Geometry: final body of the model. Coordinates: model frame, mm. Face numbers are marked on the shaded views. A direction names the side the tool comes from. Give positions to 0.01 mm unless a question says otherwise; leave off trailing zeros. Loops run counter-clockwise (first coordinate to the right, second up) from the corner with the lowest first, then second, coordinate; pieces in that order, holes last. Notation, with made-up numbers: (-15, 65.25) -> (19, 65.25) arc R14 cw to (19, 75.25) -> close; hole circle Ø8 at (16.5, 80). An arc over 180 degrees is marked (long way). Answer in a Markdown table with one row per item. Add a question column.
1) Section query B-B (z = 9.5). Return the cut outline in (x, y), plus the area to 3 significant figures.
2) Section query A-A (y = -1.5). Return the cut outline in (x, z).
3) Section query D-D (y = 8.75). Return the cut outline in (x, z).
4) Access query for the marked faces 5 and 6. Directions: +Z, -Z, +X, -X, +Y, -Y. A direction counts if a zero-diameter tool reaches every point of the face in a straight line with its end or side. Return the directions, or none.
5) Draft query along Y for the marked faces 1, 2, 3 and 4. Return one class per face: +Y half, -Y half, draft (parallel to the pull), parting line (faces both ways), or undercut.
6) Line query: line 1 (Y direction, x = 6.5, z = 14.25); line 2 (Y direction, x = -8.4, z = 5); line 3 (X direction, y = 4, z = 13). Output: solid intervals per line, ascending. Write a range as from..to.
7) First-contact query: P1, Ø0.9, axis at y = -5.5, z = 10, coming from the +X side; P2, Ø4.5, axis at y = 5, z = 15, coming from the +X side; P3, Ø6, axis at x = 8.5, y = 4.5, coming from the -Z side; P4, Ø8, axis at x = 0.5, z = 13.5, coming from the +Y side. Flat tips, straight axial feed; report the tip coordinate or a pass-through.
8) Section query C-C (y = -4.75). Return the cut outline in (x, z), plus the area to 3 significant figures.
```python
from build123d import *

# Parameters (mm, degrees)
SKETCH2_W           = 40
SKETCH2_H           = 20
BOSS_EXTRUDE2_DEPTH = 20
SKETCH3_W           = 20
SKETCH3_H           = 20
CUT_EXTRUDE1_DEPTH  = 10
SKETCH4_W           = 18.496290815
SKETCH4_H           = 3
CUT_EXTRUDE2_DEPTH  = 31
SKETCH5_R           = 1.5
CUT_EXTRUDE3_DEPTH  = 34.541019662
SKETCH8_R           = 1.5
CUT_EXTRUDE4_DEPTH  = 2.5
CUT_EXTRUDE6_DEPTH  = 31.347981811


with BuildPart() as part:
    # Sketch2 → Boss-Extrude2 (new body)
    with BuildSketch(Plane.XY):
        Rectangle(SKETCH2_W, SKETCH2_H)
    extrude(amount=BOSS_EXTRUDE2_DEPTH)

    # Sketch3 → Cut-Extrude1 (cut)
    with BuildSketch(Plane.ZY.offset(20)):
        with Locations((10, 0)):
            Rectangle(SKETCH3_W, SKETCH3_H)
    extrude(amount=-CUT_EXTRUDE1_DEPTH, mode=Mode.SUBTRACT)

    # Sketch4 → Cut-Extrude2 (cut, through all)
    with BuildSketch(Plane.XY.offset(20)):
        Polygon((-5, -1), (20, -1), (20, 0), (20, 10), (-5, 10), align=None)
        with Locations((10.751854593, -5.5)):
            Rectangle(SKETCH4_W, SKETCH4_H)
    extrude(amount=-CUT_EXTRUDE2_DEPTH, mode=Mode.SUBTRACT)

    # Sketch5 → Cut-Extrude3 (cut, through all)
    with BuildSketch(Plane(origin=(-5, 0, 0), x_dir=(0, 0, -1), z_dir=(1, 0, 0))):
        with Locations((-15.023649692, 4.5)):
            Circle(SKETCH5_R)
        with Locations((-5, 4.5)):
            Circle(SKETCH5_R)
    extrude(amount=-CUT_EXTRUDE3_DEPTH, mode=Mode.SUBTRACT)

    # Sketch8 → Cut-Extrude4 (cut)
    # profile 1 of 2: a face of its own
    with BuildSketch(Plane(origin=(-5, 0, 0), x_dir=(0, 0, -1), z_dir=(1, 0, 0))):
        Polygon((-12.208649692, 2.874758992), (-12.208649692, 6.125241008), (-15.023649692, 7.750482016), (-17.838649692, 6.125241008), (-17.838649692, 2.874758992), (-15.023649692, 1.249517984), align=None)
        with Locations((-15.023649692, 4.5)):
            Circle(SKETCH8_R, mode=Mode.SUBTRACT)
    # profile 2 of 2: a face of its own
    with BuildSketch(Plane(origin=(-5, 0, 0), x_dir=(0, 0, -1), z_dir=(1, 0, 0))):
        Polygon((-2.185, 2.874758992), (-2.185, 6.125241008), (-5, 7.750482016), (-7.815, 6.125241008), (-7.815, 2.874758992), (-5, 1.249517984), align=None)
        with Locations((-5, 4.5)):
            Circle(SKETCH8_R, mode=Mode.SUBTRACT)
    extrude(amount=-CUT_EXTRUDE4_DEPTH, mode=Mode.SUBTRACT)

    # Sketch9 → Cut-Extrude6 (cut, through all)
    with BuildSketch(Plane(origin=(0, -1, 0), x_dir=(1, 0, 0), z_dir=(0, 1, 0))):
        with BuildLine():
            ThreePointArc((11.503709185, -3.5), (10.003709185, -5), (11.503709185, -6.5))
            Line((11.503709185, -6.5), (11.503709185, -3.5))
        make_face()
        with BuildLine():
            Line((11.503709185, -3.5), (11.503709185, -6.5))
            ThreePointArc((11.503709185, -6.5), (12.564369357, -6.060660172), (13.003709185, -5))
            ThreePointArc((13.003709185, -5), (12.564369357, -3.939339828), (11.503709185, -3.5))
        make_face()
        with BuildLine():
            ThreePointArc((11.503709185, -13.5), (10.003709185, -15), (11.503709185, -16.5))
            Line((11.503709185, -16.5), (11.503709185, -13.5))
        make_face()
        with BuildLine():
            Line((11.503709185, -13.5), (11.503709185, -16.5))
            ThreePointArc((11.503709185, -16.5), (12.564369357, -16.060660172), (13.003709185, -15))
            ThreePointArc((13.003709185, -15), (12.564369357, -13.939339828), (11.503709185, -13.5))
        make_face()
    extrude(amount=-CUT_EXTRUDE6_DEPTH, mode=Mode.SUBTRACT)


solid = part.part
```
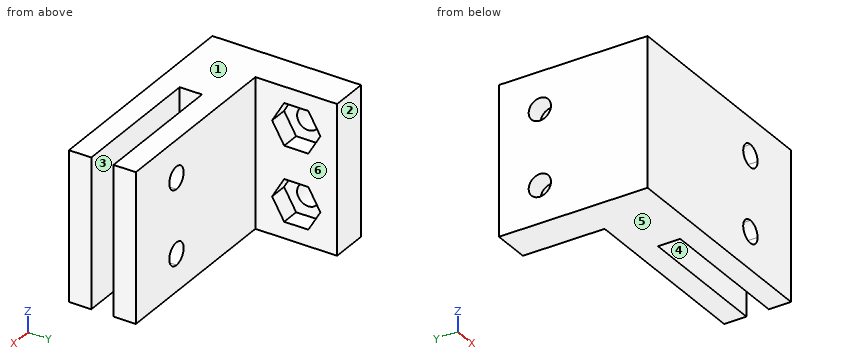
Evaluation:
| question | item | result |
|---|---|---|
| 1 | outline | (-10, -10) -> (20, -10) -> (20, -7) -> (1.5, -7) -> (1.5, -4) -> (20, -4) -> (20, -1) -> (-5, -1) -> (-5, 10) -> (-10, 10) -> close |
| 1 | area | 270 mm² |
| 2 | outline | (-10, 0) -> (20, 0) -> (20, 20) -> (-10, 20) -> close; hole circle Ø3 at (11.5, 5); hole circle Ø3 at (11.5, 15) |
| 3 | outline | (-10, 0) -> (-5, 0) -> (-5, 20) -> (-10, 20) -> close |
| 4 | face 5 | -Z, +X, -X, +Y, -Y |
| 4 | face 6 | +Z, -Z, +X, +Y |
| 5 | face 1 | draft |
| 5 | face 2 | +Y half |
| 5 | face 3 | undercut |
| 5 | face 4 | undercut |
| 6 | line 1 | -10..-7, -4..-1 |
| 6 | line 2 | -10..3, 6..10 |
| 6 | line 3 | -10..-7.5 |
| 7 | P1 | x = 1.5 |
| 7 | P2 | x = -7.5 |
| 7 | P3 | through |
| 7 | P4 | y = -1 |
| 8 | outline | (-10, 0) -> (1.5, 0) -> (1.5, 20) -> (-10, 20) -> close |
| 8 | area | 230 mm² |
